Geometry check sheet. Reference: drawing and pictorial views, mm from the part's lowest x, y, z. A direction names the side the tool comes from. Give positions to 0.01 mm unless a question says otherwise; leave off trailing zeros. Write each loop counter-clockwise with the first axis right and the second up, starting at its lowest first coordinate (ties: lowest second). Pieces come first, ordered by that corner, then holes. Notation, with made-up numbers: (16, 63) -> (59, 63) arc R30 ccw to (59, 99) -> close; hole circle Ø8 at (43.25, 77.25). An arc over 180 degrees is marked (long way). Use a Markdown table: item, result. Add a question column.
1. Cross-section at D-D (x = 39). Enter the section's corners in (y, z).
2. Release check for a two-part mould opening along X. For the marked faces 1 and 2 record: released by +X, released by -X, zero draft, split by the parting line, or undercut.
3. Cross-section at C-C (z = 2.5). Enter the section's corners in (x, y).
4. Cross-section at A-A (x = 90). Enter the section's corners in (y, z), then the cut area to 3 significant figures.
5. Set-up check for the marked faces 3, 4 and 5: record each of +Z, -Z, +X, -X, +Y, -Y from which the full face is reachable in a straight line by a thin tool's end or side.
6. Cross-section at B-B (y = 17). Enter the section's corners in (x, z) (1 decimal), then the cut area to 3 significant figures.
7. Scan lines: probe 1 along Y at (x, z) = (90, 6.75); probe 2 along Y at (x, z) = (90, 16); probe 3 along X at (y, z) = (146, 18). Record each from-to range of solid material in increasing order. Write a range as [from, to].
8. Gauge pin test, flat ends, axial feed: P1, Ø14.5, axis at x = 90, y = 143.7, coming from the -Z side; P2, Ø12, axis at y = 111, z = 6.5, coming from the -X side (1 decimal); P3, Ø10, axis at y = 55.5, z = 12.5, coming from the +X side. Record the tip position at first contact, or that the pin passes through.
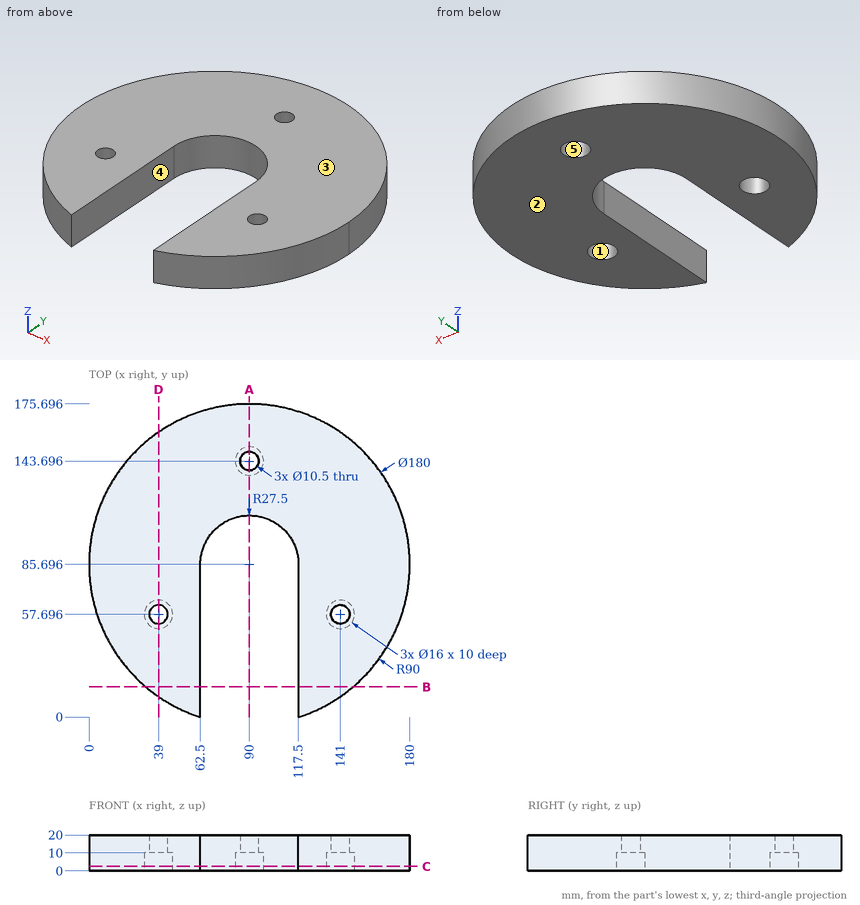
Worked answers:
| question | item | result |
|---|---|---|
| 1 | outline | (11.54, 0) -> (49.7, 0) -> (49.7, 10) -> (52.45, 10) -> (52.45, 20) -> (11.54, 20) -> close; (62.95, 10) -> (65.7, 10) -> (65.7, 0) -> (159.85, 0) -> (159.85, 20) -> (62.95, 20) -> close |
| 2 | face 1 | undercut |
| 2 | face 2 | zero draft |
| 3 | outline | (62.5, 0) -> (62.5, 85.7) arc R27.5 cw to (117.5, 85.7) -> (117.5, 0) arc R90 ccw (long way) to start; hole circle Ø16 at (39, 57.7); hole circle Ø16 at (90, 143.7); hole circle Ø16 at (141, 57.7) |
| 4 | outline | (113.2, 0) -> (135.7, 0) -> (135.7, 10) -> (138.45, 10) -> (138.45, 20) -> (113.2, 20) -> close; (148.95, 10) -> (151.7, 10) -> (151.7, 0) -> (175.7, 0) -> (175.7, 20) -> (148.95, 20) -> close |
| 4 | area | 985 mm² |
| 5 | face 3 | +Z, +X, -X, +Y, -Y |
| 5 | face 4 | +Z, -Z, -Y |
| 5 | face 5 | -Z |
| 6 | outline | (31.9, 0) -> (62.5, 0) -> (62.5, 20) -> (31.9, 20) -> close; (117.5, 0) -> (148.1, 0) -> (148.1, 20) -> (117.5, 20) -> close |
| 6 | area | 1,230 mm² |
| 7 | probe 1 | y = [113.2, 135.7], [151.7, 175.7] |
| 7 | probe 2 | y = [113.2, 138.45], [148.95, 175.7] |
| 7 | probe 3 | x = [23.19, 85.28], [94.72, 156.81] |
| 8 | P1 | stops at z = 10 |
| 8 | P2 | stops at x = 2.1 |
| 8 | P3 | stops at x = 176.4 |
